Print and shaded views of the part. All mm, measured from the part's lowest x, y and z. Round coordinates to 2 decimals unless told otherwise and drop trailing zeros. Write each loop counter-clockwise with the first axis right and the second up, starting at its lowest first coordinate (ties: lowest second). Pieces come first, ordered by that corner, then holes. Notation, with made-up numbers: (30.5, 18.5) - (78.5, 18.5) arc R18 ccw to (78.5, 38.5) - close; hole circle Ø7 at (55.25, 88.5). An arc over 180 degrees is marked (long way). One line per item, written item: value.
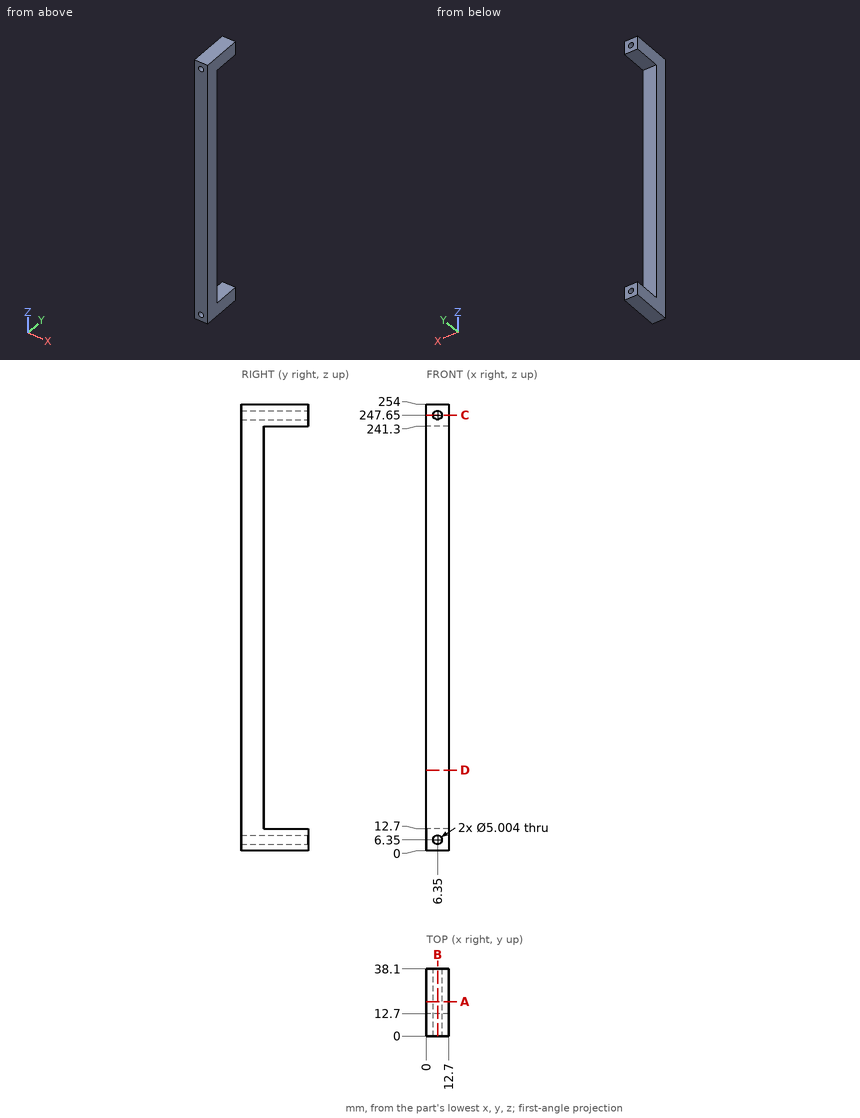
1. Wall check: probe 1 along Z at (x, y) = (6, 32); probe 2 along Z at (x, y) = (6.35, 11); probe 3 along Z at (x, y) = (6.35, 28). Give the ranges that are in metal, low to high. Write a range as [from, to].
Report:
probe 1: [0, 3.87], [8.83, 12.7], [241.3, 245.17], [250.13, 254]
probe 2: [0, 3.85], [8.85, 245.15], [250.15, 254]
probe 3: [0, 3.85], [8.85, 12.7], [241.3, 245.15], [250.15, 254]
2. Band-saw the part on A-A on y = 19.5. Write the cut outline in (x, z).
Report:
outline: (0, 0) - (12.7, 0) - (12.7, 12.7) - (0, 12.7) - close; (0, 241.3) - (12.7, 241.3) - (12.7, 254) - (0, 254) - close; hole circle Ø5 at (6.35, 6.35); hole circle Ø5 at (6.35, 247.65)
3. Band-saw the part on C-C on z = 247.65. Write the cut outline in (x, y), plus the area to 3 significant figures.
Report:
outline: (0, 0) - (3.85, 0) - (3.85, 38.1) - (0, 38.1) - close; (8.85, 0) - (12.7, 0) - (12.7, 38.1) - (8.85, 38.1) - close
area: 293 mm²
4. Band-saw the part on D-D on z = 46. Write the cut outline in (x, y), plus the area to 3 significant figures.
Report:
outline: (0, 0) - (12.7, 0) - (12.7, 12.7) - (0, 12.7) - close
area: 161 mm²
5. Drop a flat-ended pin along its axis: pin 1 (1 mm diameter, centred on x = 6, z = 176.5, fed in from +Y). Give the stop position or say it passes through.
Report:
pin 1: y = 12.7
6. Band-saw the part on B-B on x = 6.35. Write the cut outline in (y, z), plus the area to 3 significant figures.
Report:
outline: (0, 0) - (38.1, 0) - (38.1, 3.85) - (0, 3.85) - close; (0, 8.85) - (38.1, 8.85) - (38.1, 12.7) - (12.7, 12.7) - (12.7, 241.3) - (38.1, 241.3) - (38.1, 245.15) - (0, 245.15) - close; (0, 250.15) - (38.1, 250.15) - (38.1, 254) - (0, 254) - close
area: 3,490 mm²
